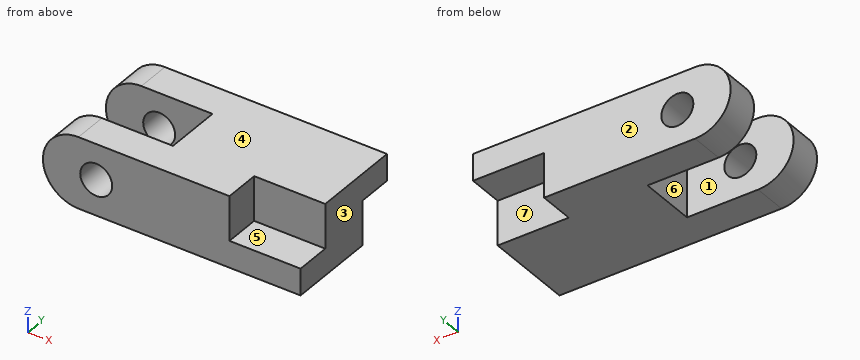
from build123d import *

# Parameters (mm, degrees)
SKETCH1_R           = 0.9
BOSS_EXTRUDE1_DEPTH = 7
CUT_EXTRUDE1_REACH  = 16.045
SKETCH2_W           = 6
SKETCH2_H           = 3.2
SKETCH3_W           = 2.5
SKETCH3_H           = 2
CUT_EXTRUDE2_DEPTH  = 4


with BuildPart() as part:
    # Sketch1 → Boss-Extrude1 (new body)
    with BuildSketch(Plane(origin=(0, 0, 0), x_dir=(1, 0, 0), z_dir=(0, 1, 0))):
        with BuildLine():
            Line((-1, 2), (11.5, 2))
            Line((11.5, 2), (11.5, -2))
            Line((11.5, -2), (-1, -2))
            ThreePointArc((-1, -2), (-3, 0), (-1, 2))
        make_face()
        with Locations(Location((0, 0, 0), (0, 0, 270))):
            Circle(SKETCH1_R, mode=Mode.SUBTRACT)
    extrude(amount=BOSS_EXTRUDE1_DEPTH)

    # Sketch2 → Cut-Extrude1 (cut, up to next)
    with BuildSketch(Plane.XY.offset(2), mode=Mode.PRIVATE) as cut_extrude1_sk1:
        with Locations((0, 3.5)):
            Rectangle(SKETCH2_W, SKETCH2_H)
    cut_extrude1_tool1 = extrude(cut_extrude1_sk1.sketch, amount=-CUT_EXTRUDE1_REACH, mode=Mode.PRIVATE) & part.part
    add(cut_extrude1_tool1.solids().sort_by_distance((0, 3.5, 2))[0], mode=Mode.SUBTRACT)

    # Sketch3 → Cut-Extrude2 (cut)
    with BuildSketch(Plane(origin=(11.5, 0, 0), x_dir=(0, 0, -1), z_dir=(1, 0, 0))):
        with Locations((0.75, 6)):
            Rectangle(SKETCH3_W, SKETCH3_H)
        with Locations((-0.75, 1)):
            Rectangle(SKETCH3_W, SKETCH3_H)
    extrude(amount=-CUT_EXTRUDE2_DEPTH, mode=Mode.SUBTRACT)


solid = part.part
Model file for the job. Use its own axes, mm. Face numbers are marked on the shaded views. A direction names the side the tool comes from. Give positions to 0.01 mm unless a question says otherwise; leave off trailing zeros. Loops run counter-clockwise (first coordinate to the right, second up) from the corner with the lowest first, then second, coordinate; pieces in that order, holes last.
1) Saw through at B-B (z = 0). Write the cut outline in (x, y), plus the area to 3 significant figures.
2) Flat gauge pins, fed straight in: pin 1 Ø1 at (x, y) = (10, 6.5) entering from -Z; pin 2 Ø2 at (x, z) = (9, 1) entering from -Y; pin 3 Ø2 at (x, z) = (-1, 0) entering from -Y; pin 4 Ø1 at (y, z) = (0.5, 1) entering from +X. Where does each tip first touch, or does it go through?
3) Pull direction Y, two halves, no side cores. Call the marked faces 1, 2 and 3: +Y half, -Y half, draft (parallel to the pull), parting line (faces both ways), or undercut.
4) Saw through at C-C (x = 10.5). Write the cut outline in (y, z), plus the area to 3 significant figures.
5) Wall check: line 1 (Z direction, x = 0, y = 5.8); line 2 (Y direction, x = 1, z = 1.2); line 3 (X direction, y = 1.35, z = 0). Give the ranges that are in metal, low to high.
6) Saw through at D-D (y = 6.5). Write the cut outline in (x, z), plus the area to 3 significant figures.
7) Saw through at A-A (x = 0). Write the cut outline in (y, z).
8) Tool access for the marked faces 4, 5, 6 and 7: list every direction of +Z, -Z, +X, -X, +Y, -Y with a clear straight run to the whole face (end or side of a thin tool).
Answer block:
1. outline: (-3, 0) - (-0.9, 0) - (-0.9, 1.9) - (-3, 1.9) - close; (-3, 5.1) - (-0.9, 5.1) - (-0.9, 7) - (-3, 7) - close; (0.9, 0) - (7.5, 0) - (7.5, 2) - (11.5, 2) - (11.5, 5) - (7.5, 5) - (7.5, 7) - (0.9, 7) - (0.9, 5.1) - (3, 5.1) - (3, 1.9) - (0.9, 1.9) - close
1. area: 59.5 mm2
2. pin 1: stops at z = 0.5
2. pin 2: stops at y = 2
2. pin 3: stops at y = 0
2. pin 4: stops at x = 7.5
3. face 1: undercut
3. face 2: +Y half
3. face 3: draft
4. outline: (0, -2) - (5, -2) - (5, 0.5) - (7, 0.5) - (7, 2) - (2, 2) - (2, -0.5) - (0, -0.5) - close
4. area: 18.0 mm2
5. line 1: z = -2 to -0.9, 0.9 to 2
5. line 2: y = 0 to 1.9, 5.1 to 7
5. line 3: x = -3 to -0.9, 0.9 to 7.5
6. outline: (-1, -2) - (7.5, -2) - (7.5, 0.5) - (11.5, 0.5) - (11.5, 2) - (-1, 2) arc R2 ccw to start; hole circle Ø1.8 at (0, 0)
6. area: 43.7 mm2
7. outline: (0, -2) - (1.9, -2) - (1.9, -0.9) - (0, -0.9) - close; (0, 0.9) - (1.9, 0.9) - (1.9, 2) - (0, 2) - close; (5.1, -2) - (7, -2) - (7, -0.9) - (5.1, -0.9) - close; (5.1, 0.9) - (7, 0.9) - (7, 2) - (5.1, 2) - close
8. face 4: +Z, +X, -X, +Y, -Y
8. face 5: +Z, +X, -Y
8. face 6: +Z, -Z, -X
8. face 7: -Z, +X, +Y
